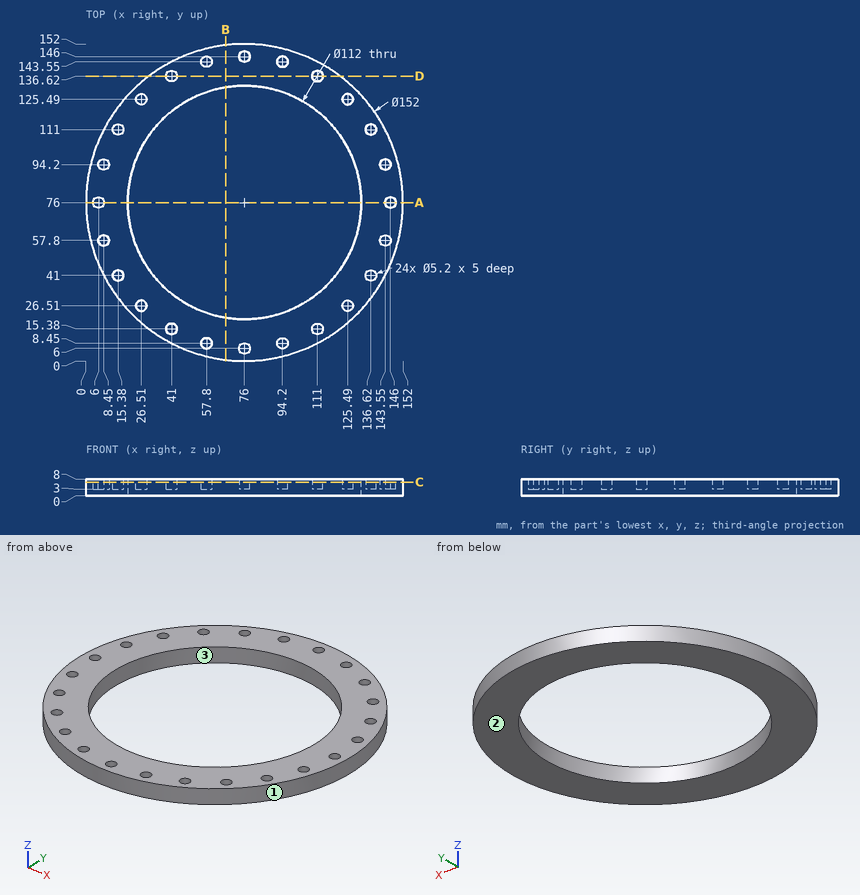
Design review of the part shown in the three views and the two pictorial views. Dimensions are in mm from the part's minimum x, y and z. Give positions to 0.01 mm unless a question says otherwise; leave off trailing zeros. Loops run counter-clockwise (first coordinate to the right, second up) from the corner with the lowest first, then second, coordinate; pieces in that order, holes last. Notation, with made-up numbers: (-18, 29.5) -> (-13, 29.5) arc R22 ccw to (-13, 64.5) -> close; hole circle Ø3 at (-38.5, 12.25). An arc over 180 degrees is marked (long way). Put each result on its own line as item: value. Start each with the question number.
1. Clearance check with flat-ended pins moving along their axes: P1, Ø6, axis at x = 16, y = 32, coming from the -Z side; P2, Ø1.6, axis at x = 59, y = 142.5, coming from the +Z side; P3, Ø8, axis at x = 87, y = 27, coming from the +Z side; P4, Ø3, axis at x = 19, z = 6.5, coming from the -Y side. State where each tip first meets the part, or that it passes through.
2. Mouldability with a two-part tool opening along X and no side actions: class the marked faces 1, 2 and 3 as released by +X, released by -X, zero draft, split by the parting line, or undercut.
3. We need section C-C on z = 6.5. State how many separate pieces and enclosed holes the cut face has, then the cut area to 3 significant figures.
4. We need section B-B on x = 67. State the section outline as (y, z) points, then the cut area to 3 significant figures.
5. We need section D-D on y = 136.62. State the section outline as (x, z) points.
6. We need section A-A on y = 76. State the section outline as (x, z) points.
7. Wall thickness on probe 1 along Y at (x, z) = (113, 5.25); probe 2 along Y at (x, z) = (16, 7.25) (3 decimals); probe 3 along X at (y, z) = (26.51, 5.2): over which ranges is each line inside the solid? List them lowest first.
Determined:
1. P1: z = 0
1. P2: z = 3
1. P3: through
1. P4: y = 24.08
2. face 1: split by the parting line
2. face 2: zero draft
2. face 3: undercut
3. separate pieces: 1
3. enclosed holes: 25
3. area: 7,780 mm^2
4. outline: (0.53, 0) -> (20.73, 0) -> (20.73, 8) -> (0.53, 8) -> close; (131.27, 0) -> (151.47, 0) -> (151.47, 8) -> (131.27, 8) -> close
4. area: 323 mm^2
5. outline: (30.16, 0) -> (121.84, 0) -> (121.84, 8) -> (113.6, 8) -> (113.6, 3) -> (108.4, 3) -> (108.4, 8) -> (43.6, 8) -> (43.6, 3) -> (38.4, 3) -> (38.4, 8) -> (30.16, 8) -> close
6. outline: (0, 0) -> (20, 0) -> (20, 8) -> (8.6, 8) -> (8.6, 3) -> (3.4, 3) -> (3.4, 8) -> (0, 8) -> close; (132, 0) -> (152, 0) -> (152, 8) -> (148.6, 8) -> (148.6, 3) -> (143.4, 3) -> (143.4, 8) -> (132, 8) -> close
7. probe 1: 9.61 to 13.72, 17.04 to 33.96, 118.04 to 134.96, 138.28 to 142.39
7. probe 2: 29.352 to 38.475, 43.525 to 108.475, 113.525 to 122.648
7. probe 3: 18.32 to 23.91, 29.11 to 49.79, 102.21 to 122.89, 128.09 to 133.68
